from build123d import *

# Parameters (mm, degrees)
BOSS_EXTRUDE1_DEPTH = 5.5
SKETCH2_W           = 30.1
SKETCH2_H           = 31.3
CUT_EXTRUDE1_DEPTH  = 1.5
SKETCH3_R           = 1.7
CUT_EXTRUDE2_DEPTH  = 38.5


with BuildPart() as part:
    # Sketch1 → Boss-Extrude1 (new body)
    with BuildSketch(Plane.XY):
        Polygon((33.8, 0), (37.5, 0), (37.5, 63), (0, 63), (0, 0), (3.7, 0), (3.7, 31.7), (33.8, 31.7), align=None)
    extrude(amount=-BOSS_EXTRUDE1_DEPTH)

    # Sketch2 → Cut-Extrude1 (cut)
    with BuildSketch(Plane.XY):
        with Locations((18.75, 47.35)):
            Rectangle(SKETCH2_W, SKETCH2_H)
    extrude(amount=-CUT_EXTRUDE1_DEPTH, mode=Mode.SUBTRACT)

    # Sketch3 → Cut-Extrude2 (cut, through all)
    with BuildSketch(Plane(origin=(37.5, 0, 0), x_dir=(0, 0, -1), z_dir=(1, 0, 0))):
        with Locations((2.75, 3.5)):
            Circle(SKETCH3_R)
        with Locations((2.75, 25.2)):
            Circle(SKETCH3_R)
    extrude(amount=-CUT_EXTRUDE2_DEPTH, mode=Mode.SUBTRACT)


solid = part.part
Build history of the part. All positions in model axes, mm. A direction names the side the tool comes from. Coordinates: 2 decimals unless noted, no trailing zeros. Write each loop counter-clockwise with the first axis right and the second up, starting at its lowest first coordinate (ties: lowest second). Pieces come first, ordered by that corner, then holes.
(1) Mould opens along Y. For faces 1 (the flat face through (0, 32, -3)), 2 (the cylindrical face through (35.676, 26.886, -2.529)), 3 (the flat face through (19, 31.7, -3)) say: pulls with the +Y half, pulls with the -Y half, needs draft (parallel to the pull), parting line crosses it, or undercut.
(2) Drill centre lines: line 1 (Y direction, x = 2.7, z = -2.75); line 2 (Z direction, x = 2, y = 25); line 3 (X direction, y = 56.5, z = -1.1). Where is each one in solid material? Low to high.
(3) Pin check, flat tips, straight feed: pin 1 Ø2 at (x, z) = (31, -3) entering from -Y; pin 2 Ø9 at (x, y) = (22, 45) entering from +Z. Stop position of each tip, or through.
(4) 3-axis set-ups, long thin cutter, end or side, ignore diameter. For faces 4 (the flat face through (19, 48, -1.5)), 5 (the flat face through (2, 0, -3)), 6 (the flat face through (33.8, 24.9, -0.9)): which of +Z, -Z, +X, -X, +Y, -Y reach the whole face in a straight line?
(5) Cut at B-B on y = 8. List the corners of the cut face in (x, z), and give its area (3 significant figures).
(6) Cut at A-A on z = -2.75. List the corners of the cut face in (x, y).
(7) Cut at C-C on y = 59. List the corners of the cut face in (x, z).
(8) Cut at D-D on x = 10. List the corners of the cut face in (y, z).
Working result:
1. face 1: needs draft
1. face 2: undercut
1. face 3: pulls with the -Y half
2. line 1: y = 0 to 1.8, 5.2 to 23.5, 26.9 to 63
2. line 2: z = -5.5 to -4.44, -1.06 to 0
2. line 3: x = 0 to 3.7, 33.8 to 37.5
3. pin 1: stops at y = 31.7
3. pin 2: stops at z = -1.5
4. face 4: +Z, +Y, -Y
4. face 5: +Z, -Z, +X, -X, -Y
4. face 6: +Z, -Y
5. outline: (0, -5.5) - (3.7, -5.5) - (3.7, 0) - (0, 0) - close; (33.8, -5.5) - (37.5, -5.5) - (37.5, 0) - (33.8, 0) - close
5. area: 40.7 mm2
6. outline: (0, 0) - (3.7, 0) - (3.7, 1.8) - (0, 1.8) - close; (0, 5.2) - (3.7, 5.2) - (3.7, 23.5) - (0, 23.5) - close; (0, 26.9) - (3.7, 26.9) - (3.7, 31.7) - (33.8, 31.7) - (33.8, 26.9) - (37.5, 26.9) - (37.5, 63) - (0, 63) - close; (33.8, 0) - (37.5, 0) - (37.5, 1.8) - (33.8, 1.8) - close; (33.8, 5.2) - (37.5, 5.2) - (37.5, 23.5) - (33.8, 23.5) - close
7. outline: (0, -5.5) - (37.5, -5.5) - (37.5, 0) - (33.8, 0) - (33.8, -1.5) - (3.7, -1.5) - (3.7, 0) - (0, 0) - close
8. outline: (31.7, -5.5) - (63, -5.5) - (63, -1.5) - (31.7, -1.5) - close
